The drawing under review shows one solid part. Ordinate dimensions are in mm from its lowest x, y, z. A direction names the side the tool comes from. Round coordinates to 2 decimals unless told otherwise and drop trailing zeros. Order: outer loops, then holes, each group sorted by start corner. A loop starts at its lowest first (then second) coordinate and runs counter-clockwise, first axis right, second up. Notation, with made-up numbers: (0, 73) -> (17, 73) arc R16 ccw to (17, 98) -> close; hole circle Ø11 at (77.25, 58.25). An arc over 180 degrees is marked (long way). Use a Markdown table: item, result. Add a question column.
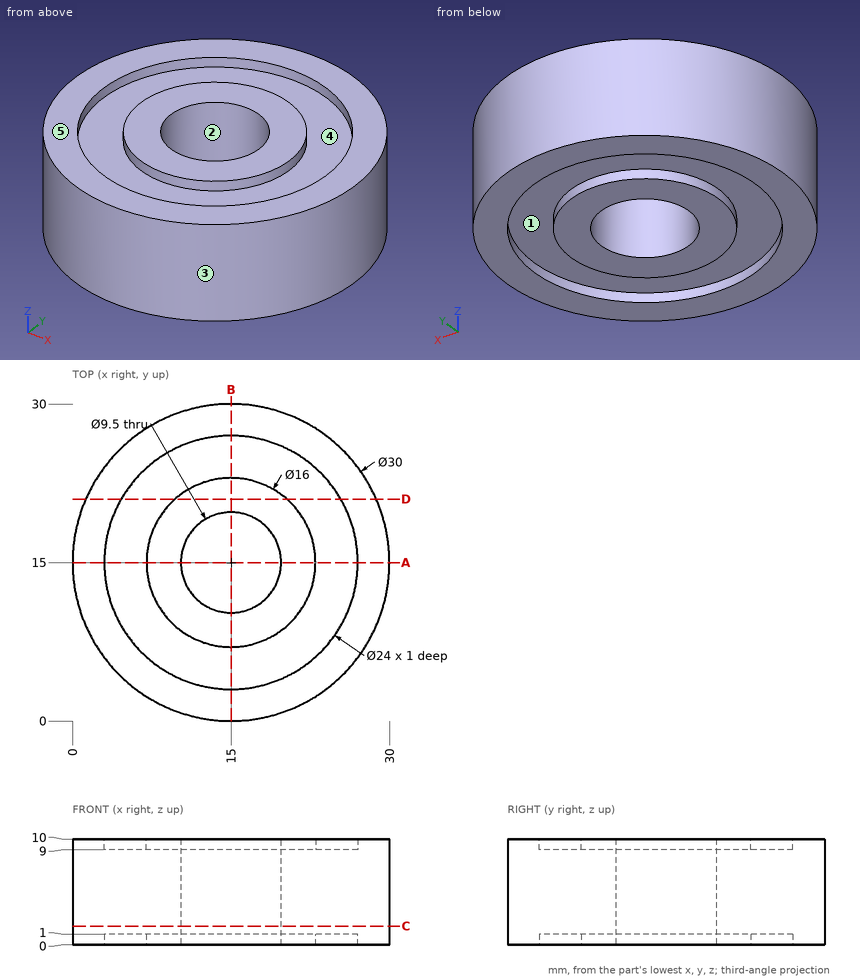
Q1. Add section D-D, the plane y = 21. Give the boundary of the cut face in (x, z), then the cut area to 3 significant figures.
Q2. Draft analysis for pull direction Y (two halves, no side actions). For the marked faces 3, 4 and 5, state which applies: released by +Y, released by -Y, zero draft, split by the parting line, or undercut.
Q3. Add section C-C, the plane z = 1.75. Give the boundary of the cut face in (x, y).
Q4. For the marked faces 1 and 2, list the 3-axis set-ups (+Z, -Z, +X, -X, +Y, -Y) from which the entire face can be reached by the end or side of a thin tool; tool diameter is ignored.
Q5. For pin 1 (6 mm diameter, centred on x = 25, z = 2, fed in from +Y); pin 2 (6 mm diameter, centred on x = 7.5, z = 2.5, fed in from -Y); pin 3 (4 mm diameter, centred on x = 23.5, z = 5.5, fed in from +Y), all flat-tipped, find the tip position at first contact; note any pin that passes through.
Q6. Add section A-A, the plane y = 15. Give the boundary of the cut face in (x, z), then the cut area to 3 significant figures.
Q7. To check wall thickness, follow line 1 along Y through (x, z) = (15, 9.4); line 2 along X through (y, z) = (14.75, 1.75); line 3 along X through (y, z) = (13.75, 3). State the ranges of each line that lie inside material, in increasing order.
Return value:
| question | item | result |
|---|---|---|
| 1 | outline | (1.25, 0) -> (4.61, 0) -> (4.61, 1) -> (9.71, 1) -> (9.71, 0) -> (20.29, 0) -> (20.29, 1) -> (25.39, 1) -> (25.39, 0) -> (28.75, 0) -> (28.75, 10) -> (25.39, 10) -> (25.39, 9) -> (20.29, 9) -> (20.29, 10) -> (9.71, 10) -> (9.71, 9) -> (4.61, 9) -> (4.61, 10) -> (1.25, 10) -> close |
| 1 | area | 255 mm² |
| 2 | face 3 | split by the parting line |
| 2 | face 4 | undercut |
| 2 | face 5 | zero draft |
| 3 | outline | circle Ø30 at (15, 15); hole circle Ø9.5 at (15, 15) |
| 4 | face 1 | -Z |
| 4 | face 2 | +Z, -Z |
| 5 | pin 1 | y = 28.27 |
| 5 | pin 2 | y = 0.69 |
| 5 | pin 3 | y = 28.52 |
| 6 | outline | (0, 0) -> (3, 0) -> (3, 1) -> (7, 1) -> (7, 0) -> (10.25, 0) -> (10.25, 10) -> (7, 10) -> (7, 9) -> (3, 9) -> (3, 10) -> (0, 10) -> close; (19.75, 0) -> (23, 0) -> (23, 1) -> (27, 1) -> (27, 0) -> (30, 0) -> (30, 10) -> (27, 10) -> (27, 9) -> (23, 9) -> (23, 10) -> (19.75, 10) -> close |
| 6 | area | 189 mm² |
| 7 | line 1 | 0 to 3, 7 to 10.25, 19.75 to 23, 27 to 30 |
| 7 | line 2 | 0 to 10.26, 19.74 to 30 |
| 7 | line 3 | 0.05 to 10.42, 19.58 to 29.95 |
